from build123d import *

# Parameters (mm, degrees)
SKETCH_1_R               = 6
EXTRUDE_1_DEPTH          = 15
SKETCH_2_R               = 3
EXTRUDE_2_DEPTH          = 20
EXTRUDE_START            = 17
SKETCH_3_R               = 3
EXTRUDE_3_DEPTH          = 17
CUT_EXTRUDE_1_DEPTH      = 10
CUT_EXTRUDE_1_DEPTH_BACK = 10
SKETCH_5_R               = 1
SKETCH_7_W               = 14.322953254
SKETCH_7_H               = 0.4
CUT_EXTRUDE_2_DEPTH      = 34


with BuildPart() as part:
    # Sketch 1 → Extrude 1 (new body)
    with BuildSketch(Plane.XY):
        Circle(SKETCH_1_R)
    extrude(amount=EXTRUDE_1_DEPTH)

    # Sketch 2 → Extrude 2 (add)
    with BuildSketch(Plane.XY.offset(15)):
        Circle(SKETCH_2_R)
    extrude(amount=EXTRUDE_2_DEPTH)

    # Sketch 3 → Extrude 3 (add)
    with BuildSketch(Plane(origin=(0, 0, 0), x_dir=(-1, 0, 0), z_dir=(0, 0, -1)).offset(EXTRUDE_START)):
        with Locations(Location((0, 0, 0), (0, 0, 180))):
            Circle(SKETCH_3_R)
    extrude(amount=-EXTRUDE_3_DEPTH)

    # Sketch 5 → Cut-Extrude 1 (cut, two sides: drawn at the far end of the back side and taken through both)
    with BuildSketch(Plane(origin=(0, 0, 0), x_dir=(1, 0, 0), z_dir=(0, 1, 0)).offset(-CUT_EXTRUDE_1_DEPTH_BACK)):
        with Locations(Location((0, -32, 0), (0, 0, 90))):
            Circle(SKETCH_5_R)
        with Locations(Location((0, 14, 0), (0, 0, 90))):
            Circle(SKETCH_5_R)
    extrude(amount=CUT_EXTRUDE_1_DEPTH + CUT_EXTRUDE_1_DEPTH_BACK, mode=Mode.SUBTRACT)

    # Sketch 7 → Cut-Extrude 2 (cut)
    with BuildSketch(Plane.XY.offset(35)):
        with Locations((-0.299039341, 0)):
            Rectangle(SKETCH_7_W, SKETCH_7_H)
    extrude(amount=-CUT_EXTRUDE_2_DEPTH, mode=Mode.SUBTRACT)


solid = part.part
The listing builds one solid part. Answer for the finished solid, in the listing's coordinates (mm). A direction names the side the tool comes from. Round coordinates to 2 decimals unless told otherwise and drop trailing zeros. Loops run counter-clockwise (first coordinate to the right, second up) from the corner with the lowest first, then second, coordinate; pieces in that order, holes last. Notation, with made-up numbers: M 78,33 L 91,33 A25 ccw 91,66 Z; hole C -27,-22 d3. An arc over 180 degrees is marked long. Write each question's results on one line, items separated by ' | '. Start each with the question number.
1) Each of these flat-tipped pins is pushed along its axis until it touches: pin 1 (1.5 mm diameter, centred on x = -1.5, z = -8, fed in from -Y); pin 2 (2.5 mm diameter, centred on x = 0, z = -14, fed in from -Y); pin 3 (3 mm diameter, centred on x = 0, z = 32, fed in from +Y). Where does it stop, or does it pass through?
2) Find section A-A on x = 0. Write down the section's boundary in (y, z).
3) Straight lines are drawn through the part: probe 1 along Y at (x, z) = (0.25, 11); probe 2 along Y at (x, z) = (2.75, 30.5); probe 3 along Z at (x, y) = (-3, -4.5). For each, find the intervals that lie inside material, in ascending order.
4) Find section D-D on x = 2.25. Write down the section's boundary in (y, z).
5) Which of the six approach directions +Z, -Z, +X, -X, +Y, -Y give full straight-line access (tool end or side, diameter ignored) to faces 5 (the cylindrical face through (0, 3, 25)), 6 (the cylindrical face through (0, -3, 25)), 7 (the flat face through (0, -0.2, 14)), 8 (the cylindrical face through (0, 0, -15)), 9 (the flat face through (-3, -1, 0))?
6) Determine the mould class of faces 1 (the flat face through (0, 0, -17)), 2 (the cylindrical face through (0, -2, 31)), 3 (the flat face through (0, 1, 35)), 4 (the cylindrical face through (0, 2, 31)) for opening direction Z: pulls with the +Z half, pulls with the -Z half, needs draft (parallel to the pull), parting line crosses it, or undercut.
Final values:
1) pin 1: y = -2.9 | pin 2: y = -3 | pin 3: y = 3
2) outline: M -6,0 L -3,0 L -3,-13 L 3,-13 L 3,0 L 6,0 L 6,15 L 3,15 L 3,31 L 0.2,31 L 0.2,1 L -0.2,1 L -0.2,31 L -3,31 L -3,15 L -6,15 Z; M -3,-17 L 3,-17 L 3,-15 L -3,-15 Z; M -3,33 L -0.2,33 L -0.2,35 L -3,35 Z; M 0.2,33 L 3,33 L 3,35 L 0.2,35 Z
3) probe 1: -5.99 to -0.2, 0.2 to 5.99 | probe 2: -1.2 to -0.2, 0.2 to 1.2 | probe 3: 0 to 15
4) outline: M -5.56,0 L -1.98,0 L -1.98,-17 L 1.98,-17 L 1.98,0 L 5.56,0 L 5.56,15 L 1.98,15 L 1.98,35 L 0.2,35 L 0.2,1 L -0.2,1 L -0.2,35 L -1.98,35 L -1.98,15 L -5.56,15 Z
5) face 5: +Z, +Y | face 6: +Z, -Y | face 7: +Z, +X, -X | face 8: +Y, -Y | face 9: -Z
6) face 1: pulls with the -Z half | face 2: undercut | face 3: pulls with the +Z half | face 4: undercut
